Model file for the job. Use its own axes, mm. Face numbers are marked on the shaded views. A direction names the side the tool comes from. Coordinates: 2 decimals unless noted, no trailing zeros. Loops run counter-clockwise (first coordinate to the right, second up) from the corner with the lowest first, then second, coordinate; pieces in that order, holes last. Notation, with made-up numbers: (-25.5, -3) - (-20.5, -3) arc R13 cw to (-20.5, 14) - close; hole circle Ø4 at (68.5, 39). An arc over 180 degrees is marked (long way). Write each question's results on one line, items separated by ' | '. Start each with the question number.
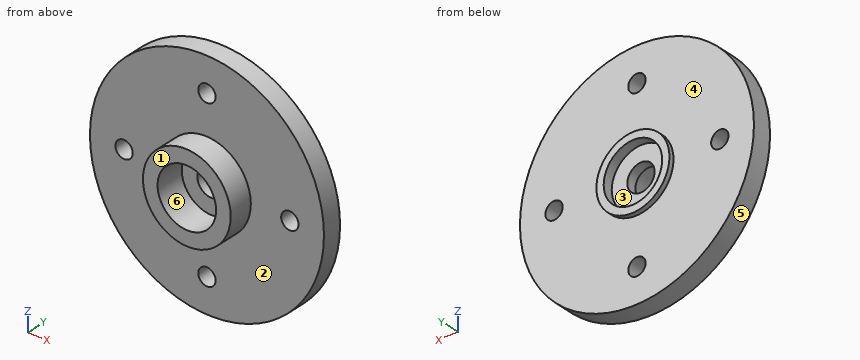
```python
from build123d import *

# Parameters (mm, degrees)
SKETCH1_W                  = 12
SKETCH1_H                  = 2
SKETCH2_R                  = 4.5
BOSS_EXTRUDE1_DEPTH        = 2.5
SKETCH3_R                  = 3.75
BOSS_EXTRUDE2_DEPTH        = 0.5
M1_6_CLEARANCE_HOLE1_D     = 1.778
M1_6_CLEARANCE_HOLE1_DEPTH = 2.5


with BuildPart() as part:
    # Sketch1 → Revolve1 (revolve)
    with BuildSketch(Plane(origin=(0, 0, 0), x_dir=(-1, 0, 0), z_dir=(0, 0, -1))):
        with Locations((38.069, 69.05714)):
            Rectangle(SKETCH1_W, SKETCH1_H)
    revolve(axis=Axis((-44.069, 68.05714, 0), (0, 1, 0)))

    # Sketch2 → Boss-Extrude1 (add)
    with BuildSketch(Plane.XZ.offset(-68.05714)):
        with Locations((-44.069, 0)):
            Circle(SKETCH2_R)
    extrude(amount=BOSS_EXTRUDE1_DEPTH)

    # Sketch3 → Boss-Extrude2 (add)
    with BuildSketch(Plane(origin=(0, 70.05714, 0), x_dir=(-1, 0, 0), z_dir=(0, 1, 0))):
        with Locations((44.069, 0)):
            Circle(SKETCH3_R)
    extrude(amount=BOSS_EXTRUDE2_DEPTH)

    # Sketch4 → Cut-Revolve1 (revolve, cut)
    with BuildSketch(Plane.XY):
        Polygon((-41.069, 70.55714), (-44.069, 70.55714), (-44.069, 65.55714), (-41.069, 65.55714), (-41.069, 68.55714), (-42.669, 68.55714), (-42.669, 69.55714), (-41.069, 69.55714), align=None)
    revolve(axis=Axis((-44.069, 70.55714, 0), (0, -1, 0)), mode=Mode.SUBTRACT)

    # M1.6 Clearance Hole1
    with Locations(Plane(origin=(0, 68.05714, 0), x_dir=(-1, 0, 0), z_dir=(0, -1, 0))):
        with Locations((44.069, 8.5), (52.569, 0), (35.569, 0), (44.069, -8.5)):
            Hole(M1_6_CLEARANCE_HOLE1_D / 2, depth=M1_6_CLEARANCE_HOLE1_DEPTH)


solid = part.part
```
Q1. Which spindle directions (+Z, -Z, +X, -X, +Y, -Y) get a long thin tool onto all of the face, cutting with end or side? Do the marked faces 1 and 2. Say none if no direction does.
Q2. Pin check, flat tips, straight feed: pin 1 (5.5 mm diameter, centred on x = -44.069, z = 0, fed in from -Y); pin 2 (1.1 mm diameter, centred on x = -52.569, z = 0, fed in from +Y); pin 3 (2 mm diameter, centred on x = -35.569, z = 0, fed in from -Y); pin 4 (1.5 mm diameter, centred on x = -50.5, y = 69, fed in from -Z). Stop position of each tip, or through.
Q3. Cut at C-C (y = 67.65). List the corners of the cut face in (x, z).
Q4. Cut at A-A (z = 0). State how many separate pieces and enclosed holes the cut face has, and give its area (3 significant figures).
Q5. Cut at D-D (z = -8.5). List the corners of the cut face in (x, y), and give its area (3 significant figures).
Q6. Drill centre lines: L1, parallel to Y at x = -48.75, z = 6; L2, parallel to X at y = 65.85, z = -2.5; L3, parallel to Z at x = -36.25, y = 68.3. Where is each one in solid material? Low to high. Write a range as from..to.
Q7. Mould opens along X. For the marked faces 3, 4, 5 and 6 say: +X half, -X half, draft (parallel to the pull), parting line (faces both ways), or undercut.
Q8. Cut at B-B (x = -46.5). List the corners of the cut face in (y, z), and give its area (3 significant figures).
Check result:
1) face 1: +Z, -Z, +X, -X, -Y | face 2: -Y
2) pin 1: y = 68.56 | pin 2: through | pin 3: y = 68.06 | pin 4: z = -10.57
3) outline: circle Ø9 at (-44.07, 0); hole circle Ø6 at (-44.07, 0)
4) separate pieces: 4 | enclosed holes: 0 | area: 40.3 mm²
5) outline: (-52.54, 68.06) - (-44.96, 68.06) - (-44.96, 70.06) - (-52.54, 70.06) - close; (-43.18, 68.06) - (-35.6, 68.06) - (-35.6, 70.06) - (-43.18, 70.06) - close | area: 30.3 mm²
6) L1: 68.06..70.06 | L2: -47.81..-45.73, -42.41..-40.33 | L3: -9.1..-0.57, 0.57..9.1
7) face 3: undercut | face 4: draft | face 5: parting line | face 6: undercut
8) outline: (65.56, -3.79) - (68.06, -3.79) - (68.06, -11.75) - (70.06, -11.75) - (70.06, -2.86) - (70.56, -2.86) - (70.56, -1.76) - (69.56, -1.76) - (69.56, 1.76) - (70.56, 1.76) - (70.56, 2.86) - (70.06, 2.86) - (70.06, 11.75) - (68.06, 11.75) - (68.06, 3.79) - (65.56, 3.79) - (65.56, 1.76) - (68.56, 1.76) - (68.56, -1.76) - (65.56, -1.76) - close | area: 54.7 mm²
